from build123d import *

# Parameters (mm, degrees)
SKETCH1_R           = 30
SKETCH1_R_2         = 9
BOSS_EXTRUDE6_DEPTH = 10
FILLET3_R           = 10


with BuildPart() as part:
    # Sketch1 → Boss-Extrude6 (new body)
    with BuildSketch(Plane.XY):
        with BuildLine():
            ThreePointArc((-6.784902735, 45.870205505), (-48.86656481, 21.950698185), (-94.721398344, 6.447687029))
            ThreePointArc((-94.721398344, 6.447687029), (-107.326810614, 3.090981083), (-120, 0))
            ThreePointArc((-120, 0), (-107.326810614, -3.090981083), (-94.721398344, -6.447687029))
            ThreePointArc((-94.721398344, -6.447687029), (-48.86656481, -21.950698185), (-6.784902735, -45.870205505))
            ThreePointArc((-6.784902735, -45.870205505), (-3.521865451, -48.147719136), (0, -50))
            ThreePointArc((0, -50), (3.521865451, -48.147719136), (6.784902735, -45.870205505))
            ThreePointArc((6.784902735, -45.870205505), (48.86656481, -21.950698185), (94.721398344, -6.447687029))
            ThreePointArc((94.721398344, -6.447687029), (107.326810614, -3.090981083), (120, 0))
            ThreePointArc((120, 0), (107.326810614, 3.090981083), (94.721398344, 6.447687029))
            ThreePointArc((94.721398344, 6.447687029), (48.86656481, 21.950698185), (6.784902735, 45.870205505))
            ThreePointArc((6.784902735, 45.870205505), (3.521865451, 48.147719136), (0, 50))
            ThreePointArc((0, 50), (-3.521865451, 48.147719136), (-6.784902735, 45.870205505))
        make_face()
        Circle(SKETCH1_R, mode=Mode.SUBTRACT)
        with Locations((-65, 0)):
            Circle(SKETCH1_R_2, mode=Mode.SUBTRACT)
        with Locations((65, 0)):
            Circle(SKETCH1_R_2, mode=Mode.SUBTRACT)
    extrude(amount=BOSS_EXTRUDE6_DEPTH)

    # Fillet3
    fillet3_edges = [part.edges().sort_by_distance(p)[0] for p in [
        (0, -50, 5),
        (120, 0, 5),
        (-120, 0, 5),
        (0, 50, 5),
    ]]
    fillet(fillet3_edges, radius=FILLET3_R)


solid = part.part
Model file for the job. Use its own axes, mm. Round coordinates to 2 decimals unless told otherwise and drop trailing zeros. Loops run counter-clockwise (first coordinate to the right, second up) from the corner with the lowest first, then second, coordinate; pieces in that order, holes last. Notation, with made-up numbers: (58, 35) -> (108, 35) arc R27 cw to (108, 63) -> close; hole circle Ø5 at (54, -6.75). An arc over 180 degrees is marked (long way). Answer as CSV lines item,"result". Start each with the question number.
1) Slice it at B-B (y = 0). State how many separate pieces and enclosed holes the cut face has, plus the area to 3 significant figures.
2) Slice it at A-A (x = 65). List the corners of the cut face in (y, z).
3) Mould opens along X. For faces 1 (the face through (-42.65, 24.84, 4.93)), 2 (the face through (-27, 15, 10)), 3 (the face through (73.584, 2.703, 4.93)), 4 (the face through (-29.97, 1.32, 4.93)) say: +X half, -X half, draft (parallel to the pull), parting line (faces both ways), or undercut.
4) Pin check, flat tips, straight feed: P1, Ø4, axis at x = 52.5, z = 2.5, coming from the +Y side; P2, Ø23.5, axis at x = -65, y = 0, coming from the -Z side; P3, Ø1.5, axis at x = -33.5, z = 3.5, coming from the +Y side; P4, Ø1.5, axis at x = -34.5, z = 3.5, coming from the +Y side. Stop position of each tip, or through.
5) Probe line 1 along X through (y, z) = (6.5, 3); line 2 along X through (y, z) = (4, 1.75); line 3 along X through (y, z) = (-23, 6). List the from-to ranges inside material, lowest first.
6) Slice it at C-C (y = 14). List the corners of the cut face in (x, z), plus the area to 3 significant figures.
Filled in:
1,separate pieces,"4"
1,enclosed holes,"0"
1,area,"837 mm2"
2,outline,"(-15.37, 0) -> (-9, 0) -> (-9, 10) -> (-15.37, 10) -> close; (9, 0) -> (15.37, 0) -> (15.37, 10) -> (9, 10) -> close"
3,face 1,"-X half"
3,face 2,"draft"
3,face 3,"undercut"
3,face 4,"undercut"
4,P1,"stops at y = 21.23"
4,P2,"stops at z = 0"
4,P3,"stops at y = 29.87"
4,P4,"stops at y = 29.34"
5,line 1,"x = -87.44 to -71.22, -58.78 to -29.29, 29.29 to 58.78, 71.22 to 87.44"
5,line 2,"x = -89 to -73.06, -56.94 to -29.73, 29.73 to 56.94, 73.06 to 89"
5,line 3,"x = -46.56 to -19.26, 19.26 to 46.56"
6,outline,"(-68.82, 0) -> (-26.53, 0) -> (-26.53, 10) -> (-68.82, 10) -> close; (26.53, 0) -> (68.82, 0) -> (68.82, 10) -> (26.53, 10) -> close"
6,area,"846 mm2"
